from build123d import *

# Parameters (mm, degrees)
F1_DEPTH = 10


with BuildPart() as f1:
    # F0 (on Top) → F1 (new body)
    with BuildSketch(Plane.XY):
        with BuildLine():
            ThreePointArc((1.59, 0), (-1.1243, 1.1243), (0, -1.59))
            ThreePointArc((0, -1.59), (1.1243, -1.1243), (1.59, 0))
        make_face()
        with BuildLine():
            ThreePointArc((15, 0), (0, 15), (-15, 0))
            Line((-15, 0), (-15, -300))
            ThreePointArc((-15, -300), (0, -315), (15, -300))
            Line((15, -300), (15, 0))
        make_face()
        with BuildLine():
            ThreePointArc((-2.5, -80), (-1.767767, -78.232233), (0, -77.5))
            ThreePointArc((0, -77.5), (1.767767, -78.232233), (2.5, -80))
            Line((2.5, -80), (2.5, -290))
            ThreePointArc((2.5, -290), (1.767767, -291.767767), (0, -292.5))
            ThreePointArc((0, -292.5), (-1.767767, -291.767767), (-2.5, -290))
            Line((-2.5, -290), (-2.5, -80))
        make_face(mode=Mode.SUBTRACT)
        with BuildLine():
            ThreePointArc((1.59, 0), (1.1243, -1.1243), (0, -1.59))
            ThreePointArc((0, -1.59), (-1.1243, 1.1243), (1.59, 0))
        make_face(mode=Mode.SUBTRACT)
    extrude(amount=F1_DEPTH)


solid = f1.part
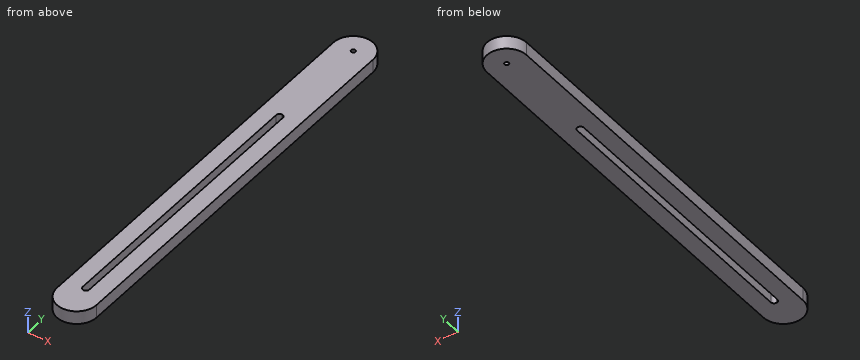
For this review, take the finished solid that the model builds, in its own axes (mm). Give positions to 0.01 mm unless a question says otherwise; leave off trailing zeros. Loops run counter-clockwise (first coordinate to the right, second up) from the corner with the lowest first, then second, coordinate; pieces in that order, holes last. Notation, with made-up numbers: M 21,-20 L 43,-20 A20 ccw 43,-7 Z; hole C 27.25,40 d5. An arc over 180 degrees is marked long. Put each result on its own line as item: value. Start each with the question number.
(1) Wall thickness on L1, parallel to X at y = -97, z = 8.5; L2, parallel to Y at x = 2, z = 5.25; L3, parallel to Y at x = -6, z = 6.5: over which ranges is each line inside the solid? List them lowest first.
(2) For pin 1 (6 mm diameter, centred on x = 6.5, z = 1.5, fed in from +Y), flat-tipped, find the tip position at first contact; note if it passes through.
(3) Add section D-D, the plane x = 11.5. Write out the cut boundary in (y, z), then the cut area to 3 significant figures.
(4) Add section B-B, the plane z = 3. Write out the cut boundary in (x, y), then the cut area to 3 significant figures.
(5) Add section C-C, the plane x = -12. Write out the cut boundary in (y, z).
(6) Add section A-A, the plane y = -181. Write out the cut boundary in (x, z).
Result:
1. L1: x = -15 to -2.5, 2.5 to 15
1. L2: y = -314.87 to -291.5, -78.5 to 14.87
1. L3: y = -313.75 to 13.75
2. pin 1: stops at y = 14.59
3. outline: M -309.63,0 L 9.63,0 L 9.63,10 L -309.63,10 Z
3. area: 3,190 mm^2
4. outline: M -15,-300 A15 ccw 15,-300 L 15,0 A15 ccw -15,0 Z; hole M -2.5,-290 A2.5 ccw 2.5,-290 L 2.5,-80 A2.5 ccw -2.5,-80 Z; hole C 0,0 d3.18
4. area: 8,630 mm^2
5. outline: M -309,0 L 9,0 L 9,10 L -309,10 Z
6. outline: M -15,0 L -2.5,0 L -2.5,10 L -15,10 Z; M 2.5,0 L 15,0 L 15,10 L 2.5,10 Z
